Drawing for the job (mm, zero at the part's lowest x, y, z). A direction names the side the tool comes from. Coordinates: 2 decimals unless noted, no trailing zeros. Write each loop counter-clockwise with the first axis right and the second up, starting at its lowest first coordinate (ties: lowest second). Pieces come first, ordered by that corner, then holes.
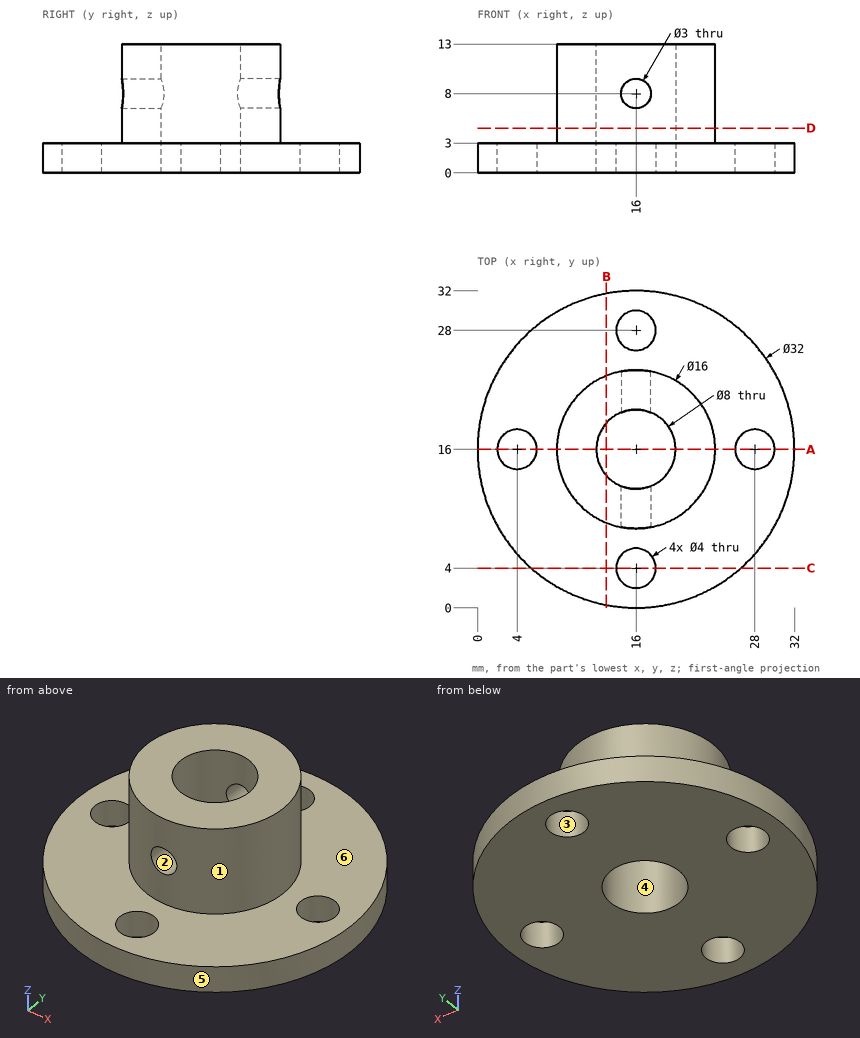
Item 1: Saw through at C-C, the plane y = 4. Write the cut outline in (x, z).
Item 2: Two-plate mould, pull along Y, no slides. Class the marked faces 1, 2, 3 and 4: +Y half, -Y half, draft (parallel to the pull), parting line (faces both ways), or undercut.
Item 3: Saw through at A-A, the plane y = 16. Write the cut outline in (x, z), and give its area (3 significant figures).
Item 4: Which spindle directions (+Z, -Z, +X, -X, +Y, -Y) get a long thin tool onto all of the face, cutting with end or side? Do the marked faces 5 and 6. Say none if no direction does.
Item 5: Saw through at B-B, the plane x = 13. Write the cut outline in (y, z).
Item 6: Wall check: line 1 along Y through (x, z) = (16, 1.35); line 2 along Z through (x, y) = (30, 17); line 3 along Y through (x, z) = (19, 5.25). Give the ranges that are in metal, low to high.
Item 7: Flat gauge pins, fed straight in: pin 1 Ø5 at (x, y) = (6.5, 23) entering from +Z; pin 2 Ø1 at (x, z) = (9, 4.5) entering from +Y; pin 3 Ø1.5 at (x, z) = (3.5, 3.5) entering from -Y. Where does each tip first touch, or does it go through?
Item 8: Saw through at D-D, the plane z = 4.5. Write the cut outline in (x, y).
Working result:
1. outline: (5.42, 0) - (14, 0) - (14, 3) - (5.42, 3) - close; (18, 0) - (26.58, 0) - (26.58, 3) - (18, 3) - close
2. face 1: parting line
2. face 2: draft
2. face 3: undercut
2. face 4: undercut
3. outline: (0, 0) - (2, 0) - (2, 3) - (0, 3) - close; (6, 0) - (12, 0) - (12, 13) - (8, 13) - (8, 3) - (6, 3) - close; (20, 0) - (26, 0) - (26, 3) - (24, 3) - (24, 13) - (20, 13) - close; (30, 0) - (32, 0) - (32, 3) - (30, 3) - close
3. area: 128 mm2
4. face 5: +Z, -Z
4. face 6: +Z
5. outline: (0.28, 0) - (13.35, 0) - (13.35, 13) - (8.58, 13) - (8.58, 3) - (0.28, 3) - close; (18.65, 0) - (31.72, 0) - (31.72, 3) - (23.42, 3) - (23.42, 13) - (18.65, 13) - close
6. line 1: y = 0 to 2, 6 to 12, 20 to 26, 30 to 32
6. line 2: z = 0 to 3
6. line 3: y = 8.58 to 13.35, 18.65 to 23.42
7. pin 1: stops at z = 3
7. pin 2: stops at y = 20.66
7. pin 3: stops at y = 5.35
8. outline: circle Ø16 at (16, 16); hole circle Ø8 at (16, 16)
